For this review, take the finished solid that the model builds, in its own axes (mm). Face numbers are marked on the shaded views. A direction names the side the tool comes from. Give positions to 0.01 mm unless a question says otherwise; leave off trailing zeros. Order: outer loops, then holes, each group sorted by start corner. A loop starts at its lowest first (then second) coordinate and runs counter-clockwise, first axis right, second up. Notation, with made-up numbers: (-22.75, 78) -> (5.25, 78) arc R21 cw to (5.25, 86) -> close; hole circle Ø8 at (64.25, 60). An arc over 180 degrees is marked (long way). One line per item, written item: value. Start each with the question number.
from build123d import *

# Parameters (mm, degrees)
SKETCH1_W           = 35.4
SKETCH1_H           = 19.293489948
BOSS_EXTRUDE1_DEPTH = 3
SKETCH1_2_W         = 35.4
SKETCH1_2_H         = 19.293489948
BOSS_EXTRUDE2_DEPTH = 3


with BuildPart() as part:
    # Sketch1 → Boss-Extrude1 (new body)
    with BuildSketch(Plane(origin=(0, 0, 0), x_dir=(1, 0, 0), z_dir=(0, 1, 0))):
        with Locations((-0.2, -3.182643359)):
            Rectangle(SKETCH1_W, SKETCH1_H)
        Polygon((-8.9, -1.732050808), (-8.9, 1.732050808), (-11.9, 3.464101615), (-14.9, 1.732050808), (-14.9, -1.732050808), (-11.9, -3.464101615), align=None, mode=Mode.SUBTRACT)
        Polygon((-1, -1.703183294), (-1, 1.703183294), (-3.95, 3.406366588), (-6.9, 1.703183294), (-6.9, -1.703183294), (-3.95, -3.406366588), align=None, mode=Mode.SUBTRACT)
        Polygon((6.8, -1.674315781), (6.8, 1.674315781), (3.9, 3.348631561), (1, 1.674315781), (1, -1.674315781), (3.9, -3.348631561), align=None, mode=Mode.SUBTRACT)
        Polygon((14.5, -1.645448267), (14.5, 1.645448267), (11.65, 3.290896534), (8.8, 1.645448267), (8.8, -1.645448267), (11.65, -3.290896534), align=None, mode=Mode.SUBTRACT)
        Polygon((-7.925, -3.420800345), (-10.725, -5.037381099), (-10.725, -8.270542606), (-7.925, -9.88712336), (-5.125, -8.270542606), (-5.125, -5.037381099), align=None, mode=Mode.SUBTRACT)
        Polygon((7.925, -3.536270399), (5.225, -5.095116126), (5.225, -8.212807579), (7.925, -9.771653306), (10.625, -8.212807579), (10.625, -5.095116126), align=None, mode=Mode.SUBTRACT)
        Polygon((0, -3.478535372), (-2.75, -5.066248612), (-2.75, -8.241675093), (0, -9.829388333), (2.75, -8.241675093), (2.75, -5.066248612), align=None, mode=Mode.SUBTRACT)
    extrude(amount=BOSS_EXTRUDE1_DEPTH)

    # Sketch1<2> → Boss-Extrude2 (add)
    with BuildSketch(Plane(origin=(0, 0, 0), x_dir=(1, 0, 0), z_dir=(0, 1, 0))):
        with Locations((-0.2, -3.182643359)):
            Rectangle(SKETCH1_2_W, SKETCH1_2_H)
    extrude(amount=-BOSS_EXTRUDE2_DEPTH)


solid = part.part
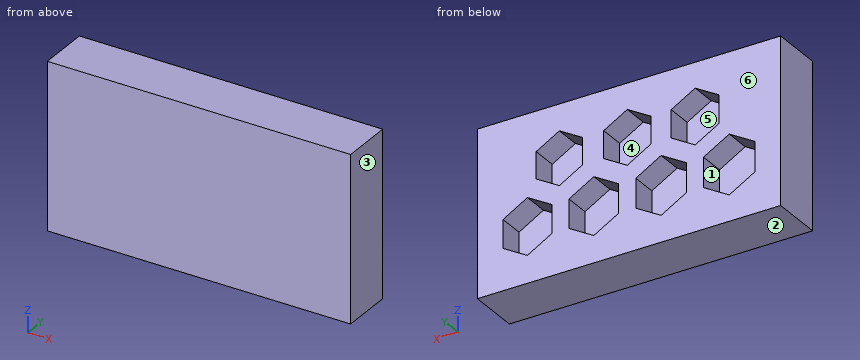
Q1. Take a section at C-C (y = 2.6). State how many separate pieces and enclosed holes the cut face has, and give its area (3 significant figures).
Q2. Take a section at D-D (z = 1). State the section outline as (x, y) points.
Q3. For line 1 along X through (y, z) = (2.25, 5.25) (3 decimals); line 2 along X through (y, z) = (1.6, -0.5); line 3 along Z through (x, y) = (-9, 2.65), list the stretches that pass through material, from the lowest coordinate up.
Q4. For the marked faces 5 and 6, list the 3-axis set-ups (+Z, -Z, +X, -X, +Y, -Y) from which the entire face can be reached by the end or side of a thin tool; tool diameter is ignored.
Q5. For pin 1 Ø3 at (x, z) = (-0.5, 7.5) entering from +Y, flat-tipped, find the tip position at first contact; note if it passes through.
Q6. Take a section at B-B (x = -13.5). State the section outline as (y, z) points.
Q7. Mouldability with a two-part tool opening along X and no side actions: class the marked faces 1, 2, 3 and 4 as pulls with the +X half, pulls with the -X half, needs draft (parallel to the pull), parting line crosses it, or undercut.
Q8. Take a section at A-A (z = 5.75). State the section outline as (x, y) points (3 decimals), and give its area (3 significant figures).
Answers below:
1. separate pieces: 1
1. enclosed holes: 7
1. area: 486 mm²
2. outline: (-17.9, -3) -> (17.5, -3) -> (17.5, 3) -> (14.5, 3) -> (14.5, 0) -> (8.8, 0) -> (8.8, 3) -> (6.8, 3) -> (6.8, 0) -> (1, 0) -> (1, 3) -> (-1, 3) -> (-1, 0) -> (-6.9, 0) -> (-6.9, 3) -> (-8.9, 3) -> (-8.9, 0) -> (-14.9, 0) -> (-14.9, 3) -> (-17.9, 3) -> close
3. line 1: x = -17.9 to -10.725, -5.125 to -2.75, 2.75 to 5.225, 10.625 to 17.5
3. line 2: x = -17.9 to -14.9, -8.9 to -6.9, -1 to 1, 6.8 to 8.8, 14.5 to 17.5
3. line 3: z = -6.46 to -1.79, 1.79 to 4.04, 9.27 to 12.83
4. face 5: +Y
4. face 6: +Z, -Z, +X, -X, +Y
5. pin 1: stops at y = 0
6. outline: (-3, -6.46) -> (3, -6.46) -> (3, -2.54) -> (0, -2.54) -> (0, 2.54) -> (3, 2.54) -> (3, 12.83) -> (-3, 12.83) -> close
7. face 1: undercut
7. face 2: needs draft
7. face 3: pulls with the +X half
7. face 4: undercut
8. outline: (-17.9, -3) -> (17.5, -3) -> (17.5, 3) -> (10.625, 3) -> (10.625, 0) -> (5.225, 0) -> (5.225, 3) -> (2.75, 3) -> (2.75, 0) -> (-2.75, 0) -> (-2.75, 3) -> (-5.125, 3) -> (-5.125, 0) -> (-10.725, 0) -> (-10.725, 3) -> (-17.9, 3) -> close
8. area: 163 mm²
